```python
from build123d import *

# Parameters (mm, degrees)
BOSS_EXTRUDE1_DEPTH = 104.45
SKETCH2_R           = 3.25
CUT_EXTRUDE1_DEPTH  = 946.639382904


with BuildPart() as part:
    # Sketch1 → Boss-Extrude1 (new body)
    with BuildSketch(Plane(origin=(0, 0, 0), x_dir=(1, 0, 0), z_dir=(0, 1, 0))):
        Polygon((916.4, 30.468956062), (23.4, 30.468956062), (23.4, 40.468956062), (0, 40.468956062), (0, 42.468956062), (25.4, 42.468956062), (25.4, 32.468956062), (914.4, 32.468956062), (914.4, 42.468956062), (939.8, 42.468956062), (939.8, 40.468956062), (916.4, 40.468956062), align=None)
    extrude(amount=BOSS_EXTRUDE1_DEPTH)

    # Sketch2 → Cut-Extrude1 (cut, through all)
    with BuildSketch(Plane.XY.offset(-40.468956062)):
        with Locations((927.1, 11.11)):
            Circle(SKETCH2_R)
        with Locations((927.1, 93.34)):
            Circle(SKETCH2_R)
        with Locations((12.7, 11.11)):
            Circle(SKETCH2_R)
        with Locations((12.7, 93.34)):
            Circle(SKETCH2_R)
    extrude(amount=-CUT_EXTRUDE1_DEPTH, mode=Mode.SUBTRACT)


solid = part.part
```
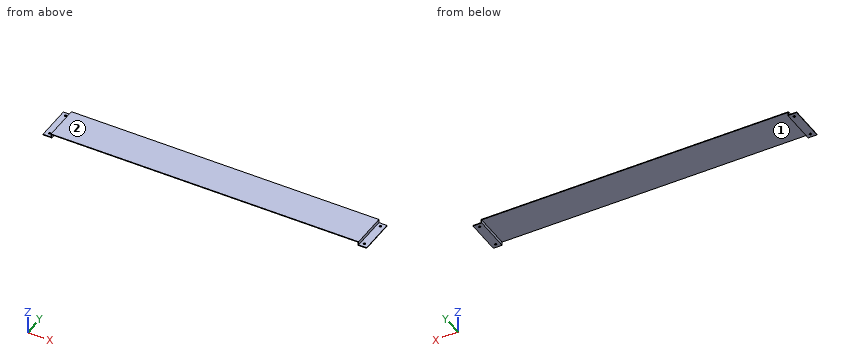
Geometry: final body of the model. Coordinates: model frame, mm. Face numbers are marked on the shaded views. Coordinates: 2 decimals unless noted, no trailing zeros. Order: outer loops, then holes, each group sorted by start corner. A loop starts at its lowest first (then second) coordinate and runs counter-clockwise, first axis right, second up. Notation, with made-up numbers: (8.5, -11) - (21.5, -11) arc R28 cw to (21.5, 8) - close; hole circle Ø1 at (44, -1). An arc over 180 degrees is marked (long way). Write each question's results on one line, items separated by ' | '.
(1) Section query C-C, the plane x = 443.5. Return the cut outline in (y, z), plus the area to 3 significant figures.
Values found:
outline: (0, -32.47) - (104.45, -32.47) - (104.45, -30.47) - (0, -30.47) - close | area: 209 mm²
(2) Section query A-A, the plane z = -38.5. Return the cut outline in (x, y).
Values found:
outline: (23.4, 0) - (25.4, 0) - (25.4, 104.45) - (23.4, 104.45) - close; (914.4, 0) - (916.4, 0) - (916.4, 104.45) - (914.4, 104.45) - close
(3) Mould query, pull axis X, two halves, no side actions, for the marked faces 1 and 2. Classes: +X half, -X half, draft (parallel to the pull), parting line (faces both ways), or undercut.
Values found:
face 1: undercut | face 2: draft
(4) Line query: line 1 (Y direction, x = 12.7, z = -41.1); line 2 (X direction, y = 47.5, z = -39); line 3 (Z direction, x = 312.5, y = 25.5). Output: solid intervals per line, ascending. Write a range as [from, to].
Values found:
line 1: y = [0, 7.86], [14.36, 90.09], [96.59, 104.45] | line 2: x = [23.4, 25.4], [914.4, 916.4] | line 3: z = [-32.47, -30.47]
(5) First-contact query: pin 1 Ø1 at (y, z) = (59, -37) entering from -X; pin 2 Ø5 at (y, z) = (77, -37) entering from +X; pin 3 Ø11.5 at (x, y) = (928, 52) entering from +Z. Flat tips, straight axial feed; report the tip coordinate or a pass-through.
Values found:
pin 1: stops at x = 23.4 | pin 2: stops at x = 916.4 | pin 3: stops at z = -40.47
(6) Section query B-B, the plane y = 29.5. Return the cut outline in (x, z), plus the area to 3 significant figures.
Values found:
outline: (0, -42.47) - (25.4, -42.47) - (25.4, -32.47) - (914.4, -32.47) - (914.4, -42.47) - (939.8, -42.47) - (939.8, -40.47) - (916.4, -40.47) - (916.4, -30.47) - (23.4, -30.47) - (23.4, -40.47) - (0, -40.47) - close | area: 1,920 mm²
